Geometry check sheet. Reference: drawing and pictorial views, mm from the part's lowest x, y, z. Give positions to 0.01 mm unless a question says otherwise; leave off trailing zeros. Order: outer loops, then holes, each group sorted by start corner. A loop starts at its lowest first (then second) coordinate and runs counter-clockwise, first axis right, second up.
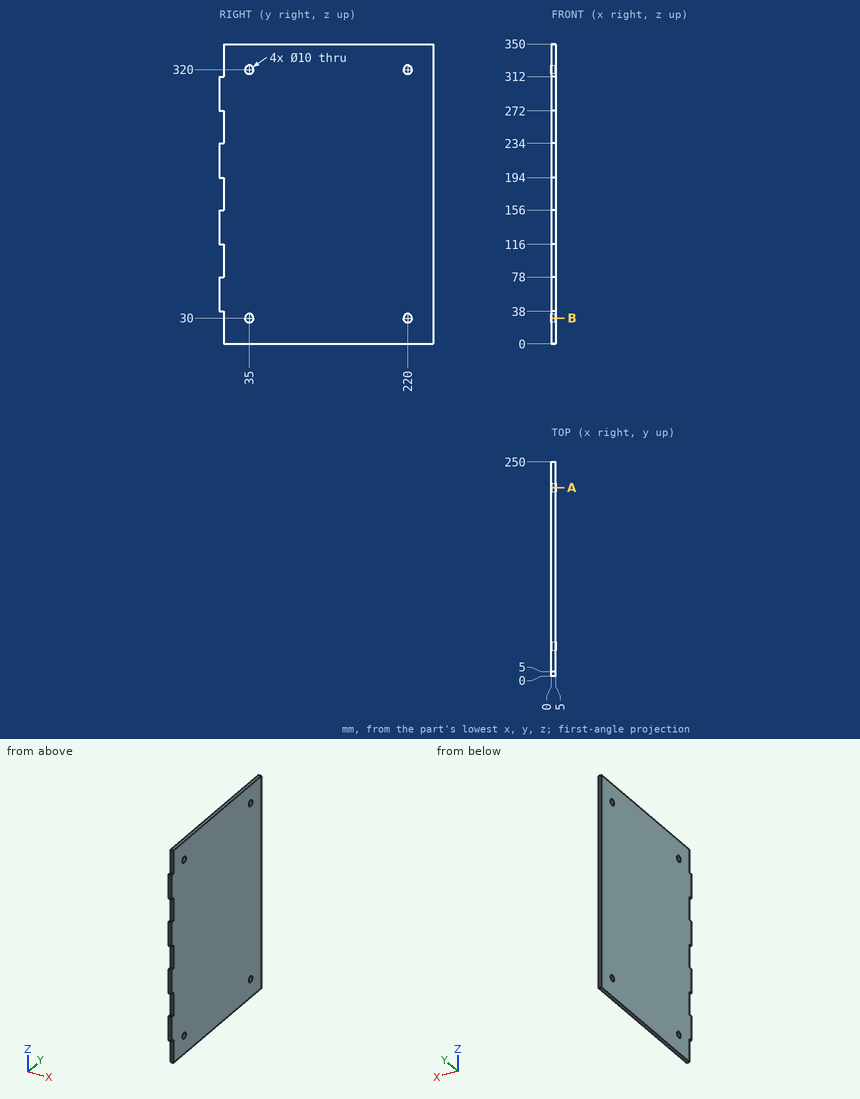
(1) Sectioned sample at A-A (y = 220). Enter the section's corners in (x, z).
(2) Go/stop test with flat-tipped pins: P1, Ø2.5, axis at x = 2, y = 3.5, coming from the -Z side; P2, Ø10, axis at y = 112.5, z = 173.5, coming from the -X side; P3, Ø9, axis at y = 35, z = 30, coming from the +X side; P4, Ø1.5, axis at x = 1.5, y = 1.5, coming from the +Z side. Record where each tip stops, or that it passes through.
(3) Sectioned sample at B-B (z = 30). Enter the section's corners in (x, y).
(4) Thickness scan on L1, parallel to Y at x = 1.4, z = 30; L2, parallel to Y at x = 0.9, z = 317; L3, parallel to Z at x = 4.1, y = 223. Record the ranges inside material, lowest first.
Values follow:
1. outline: (0, 0) - (5, 0) - (5, 25) - (0, 25) - close; (0, 35) - (5, 35) - (5, 315) - (0, 315) - close; (0, 325) - (5, 325) - (5, 350) - (0, 350) - close
2. P1: stops at z = 38
2. P2: stops at x = 0
2. P3: passes through
2. P4: stops at z = 312
3. outline: (0, 5) - (5, 5) - (5, 30) - (0, 30) - close; (0, 40) - (5, 40) - (5, 215) - (0, 215) - close; (0, 225) - (5, 225) - (5, 250) - (0, 250) - close
4. L1: y = 5 to 30, 40 to 215, 225 to 250
4. L2: y = 5 to 31, 39 to 216, 224 to 250
4. L3: z = 0 to 26, 34 to 316, 324 to 350
